```python
from build123d import *

# Parameters (mm, degrees)
F0_W     = 5.5
F0_H     = 21
F0_R     = 3.6
F0_R_2   = 2.2
F1_DEPTH = 5


with BuildPart() as f1:
    # F0 (on Top) → F1 (new body)
    with BuildSketch(Plane.XY):
        with BuildLine():
            ThreePointArc((10.08, 75), (7.151068, 82.071068), (0.08, 85))
            Line((0.08, 85), (-0.08, 85))
            ThreePointArc((-0.08, 85), (-7.151068, 82.071068), (-10.08, 75))
            Line((-10.08, 75), (-10.08, -75))
            ThreePointArc((-10.08, -75), (-7.151068, -82.071068), (-0.08, -85))
            Line((-0.08, -85), (10.08, -85))
            Line((10.08, -85), (19.920046, -85))
            ThreePointArc((19.920046, -85), (23.455545, -83.535569), (24.920046, -80.0001))
            Line((24.920046, -80.0001), (24.92016, -74.339954))
            ThreePointArc((24.92016, -74.339954), (24.92, -74.2999), (24.920161, -74.259846))
            ThreePointArc((24.920161, -74.259846), (29.940077, -69.30004), (34.92, -74.3))
            Line((34.92, -74.3), (34.92, -124))
            ThreePointArc((34.92, -124), (36.677359, -128.242641), (40.92, -130))
            ThreePointArc((40.92, -130), (45.162641, -128.242641), (46.92, -124))
            Line((46.92, -124), (46.92, -64.84))
            ThreePointArc((46.92, -64.84), (43.991068, -57.768932), (36.92, -54.84))
            Line((36.92, -54.84), (34.92, -54.84))
            Line((34.92, -54.84), (20.08, -54.84))
            ThreePointArc((20.08, -54.84), (13.008932, -51.911068), (10.08, -44.84))
            Line((10.08, -44.84), (10.08, 75))
        make_face()
        with Locations((-5.08, -40)):
            Rectangle(F0_W, F0_H, mode=Mode.SUBTRACT)
        with Locations((5, -69.92)):
            Circle(F0_R, mode=Mode.SUBTRACT)
        with Locations((40.92, -124)):
            Circle(F0_R_2, mode=Mode.SUBTRACT)
        with Locations((40.92, -74.3)):
            Circle(F0_R_2, mode=Mode.SUBTRACT)
        with Locations((-5.08, 10)):
            Rectangle(F0_W, F0_H, mode=Mode.SUBTRACT)
        with Locations((-5.08, 60)):
            Rectangle(F0_W, F0_H, mode=Mode.SUBTRACT)
    extrude(amount=F1_DEPTH)


solid = f1.part
```
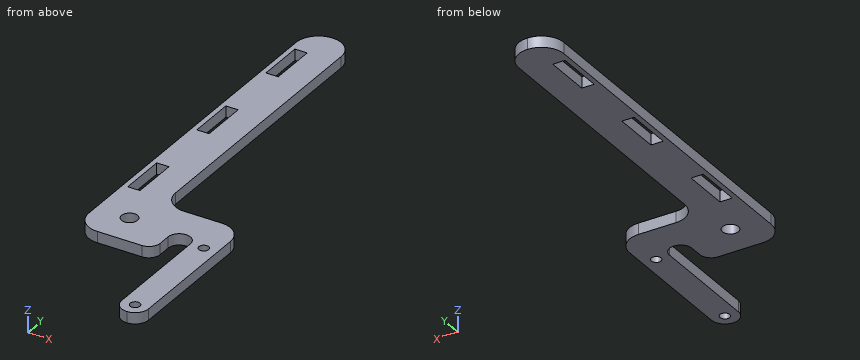
Can you work these out from the model? Positions are in its coordinate system, mm. Give positions to 0.01 mm unless a question says otherwise; leave off trailing zeros. Loops run counter-clockwise (first coordinate to the right, second up) from the corner with the lowest first, then second, coordinate; pieces in that order, holes last. Notation, with made-up numbers: M 3.25,77.25 L 14.25,77.25 A27 cw 14.25,103.25 Z; hole C -19.75,11.5 d6. An arc over 180 degrees is marked long. One line per question, with ' | ' between items. Start each with the question number.
Q1. If we section it at C-C (x = -6): Please give me the cut outline in (y, z), plus the area to 3 significant figures.
Q2. For pin 1 Ø1.5 at (y, z) = (31.5, 1.5) entering from +X; pin 2 Ø2.5 at (x, z) = (-4.5, 3.5) entering from +Y; pin 3 Ø2.5 at (x, y) = (40.92, -124) entering from -Z; pin 4 Ø3 at (x, z) = (35, 3.5) entering from +Y, each with a flat end and sliding along its axis, tell me the tip position at first contact or that it passes through.
Q3. If we section it at B-B (z = 2.35): State how many separate pieces and enclosed holes the cut face has, plus the area to 3 significant figures.
Q4. If I drill on line 1 (Y direction, x = 40.92, z = 1.3); line 2 (Y direction, x = -6.5, z = 3.25); line 3 (X direction, y = 20, z = 0.7), over which ranges is the centre line in solid material (lowest first)? Write a range as from..to.
Q5. If we section it at D-D (x = 5): Please give me the cut outline in (y, z).
Q6. If we section it at A-A (y = 6.5): Please give me the cut outline in (x, z), plus the area to 3 significant figures.
Computed:
1) outline: M -83.06,0 L -50.5,0 L -50.5,5 L -83.06,5 Z; M -29.5,0 L -0.5,0 L -0.5,5 L -29.5,5 Z; M 20.5,0 L 49.5,0 L 49.5,5 L 20.5,5 Z; M 70.5,0 L 83.06,0 L 83.06,5 L 70.5,5 Z | area: 516 mm²
2) pin 1: stops at x = 10.08 | pin 2: stops at y = 84.48 | pin 3: passes through | pin 4: stops at y = -54.84
3) separate pieces: 1 | enclosed holes: 6 | area: 4,430 mm²
4) line 1: y = -130..-126.2, -121.8..-76.5, -72.1..-55.67 | line 2: y = -82.67..-50.5, -29.5..-0.5, 20.5..49.5, 70.5..82.67 | line 3: x = -10.08..-7.83, -2.33..10.08
5) outline: M -85,0 L -73.52,0 L -73.52,5 L -85,5 Z; M -66.32,0 L 83.71,0 L 83.71,5 L -66.32,5 Z
6) outline: M -10.08,0 L -7.83,0 L -7.83,5 L -10.08,5 Z; M -2.33,0 L 10.08,0 L 10.08,5 L -2.33,5 Z | area: 73.3 mm²
